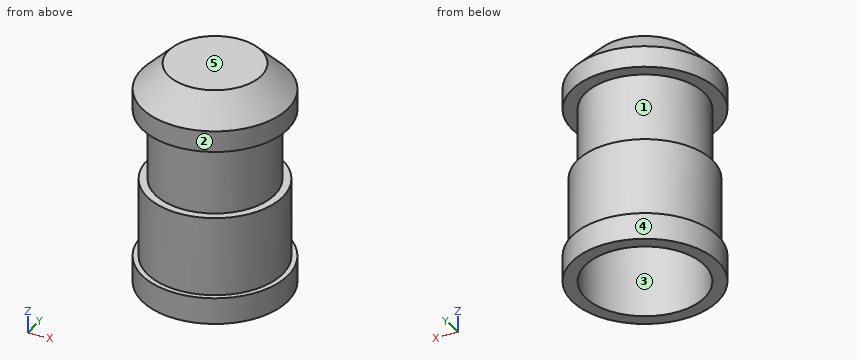
```python
from build123d import *

# Parameters (mm, degrees)
F0_R          = 2.55
F0_R_2        = 2.25
F1_DEPTH      = 4
F2_START      = -3
F0_R_3        = 2.75
F2_DEPTH      = 1
F3_DEPTH      = 4.5
F3_DEPTH_BACK = 1
F4_START      = 2.7
F4_DEPTH      = 1.8
F5_SIZE       = 1


with BuildPart() as f1:
    # F0 (on Top) → F1 (new body)
    with BuildSketch(Plane.XY):
        Circle(F0_R)
        Circle(F0_R_2, mode=Mode.SUBTRACT)
    extrude(amount=-F1_DEPTH)

    # F0 (on Top) → F2 (join)
    with BuildSketch(Plane.XY.offset(F2_START)):
        Circle(F0_R_3)
        Circle(F0_R, mode=Mode.SUBTRACT)
    extrude(amount=-F2_DEPTH)

    # F0 (on Top) → F3 (join, two sides)
    with BuildSketch(Plane.XY) as f3_sk:
        Circle(F0_R_2)
    extrude(amount=F3_DEPTH)
    extrude(f3_sk.sketch, amount=-F3_DEPTH_BACK)

    # F0 (on Top) → F4 (join)
    with BuildSketch(Plane.XY.offset(F4_START)):
        Circle(F0_R_3)
        Circle(F0_R, mode=Mode.SUBTRACT)
        Circle(F0_R)
        Circle(F0_R_2, mode=Mode.SUBTRACT)
    extrude(amount=F4_DEPTH)

    # F5
    f5_edges = [f1.edges().sort_by_distance(p)[0] for p in [
        (-2.75, 0, 4.5),
    ]]
    chamfer(f5_edges, length=F5_SIZE)


solid = f1.part
```
Work out the finished part from the listing and answer in its coordinate system (mm). Face numbers are marked on the shaded views. A direction names the side the tool comes from. Give positions to 0.01 mm unless a question says otherwise; leave off trailing zeros. Write each loop counter-clockwise with the first axis right and the second up, starting at its lowest first coordinate (ties: lowest second). Pieces come first, ordered by that corner, then holes. Notation, with made-up numbers: (-37.75, -40) -> (-28.75, -40) arc R7 ccw to (-28.75, -30) -> close; hole circle Ø7 at (66, -22). An arc over 180 degrees is marked (long way). Write item = value, one per line.
Q1. Section A-A on y = 0 is taken. Determine the outline of the cut face in (x, z), and give its area (4 significant figures).
Computed values:
outline = (-2.75, -4) -> (-2.25, -4) -> (-2.25, -1) -> (2.25, -1) -> (2.25, -4) -> (2.75, -4) -> (2.75, -3) -> (2.55, -3) -> (2.55, 0) -> (2.25, 0) -> (2.25, 2.7) -> (2.75, 2.7) -> (2.75, 3.5) -> (1.75, 4.5) -> (-1.75, 4.5) -> (-2.75, 3.5) -> (-2.75, 2.7) -> (-2.25, 2.7) -> (-2.25, 0) -> (-2.55, 0) -> (-2.55, -3) -> (-2.75, -3) -> close
area = 28.35 mm^2
Q2. A tool of negligible diameter and unlimited length cuts with its end or side. For the marked faces 1 and 2, from which of +Z, -Z, +X, -X, +Y, -Y can it reach the whole face along a straight path? Write none if from no direction.
Computed values:
face_1 = none
face_2 = +Z, -Z
Q3. Section D-D on z = -2 is taken. Determine the outline of the cut face in (x, y), and give its area (3 significant figures).
Computed values:
outline = circle Ø5.1 at (0, 0); hole circle Ø4.5 at (0, 0)
area = 4.52 mm^2
Q4. Section C-C on z = 2.25 is taken. Determine the outline of the cut face in (x, y).
Computed values:
outline = circle Ø4.5 at (0, 0)
Q5. For a pull along Y with two mould halves and no side action, classify the marked faces 3, 4 and 5 as pulls with the +Y half, pulls with the -Y half, needs draft (parallel to the pull), parting line crosses it, or undercut.
Computed values:
face_3 = undercut
face_4 = parting line crosses it
face_5 = needs draft
Q6. Flat-ended cylindrical pins translate along their axes: pin 1 Ø1.3 at (x, y) = (0.5, 0.5) entering from -Z; pin 2 Ø1 at (x, z) = (-2, 3.5) entering from -Y. Find the tip coordinate at first contact, or state that the pin passes through.
Computed values:
pin_1 = -1
pin_2 = -2.3
Q7. Consider line 1 along X through (y, z) = (-0.5, -1.5); line 2 along Y through (x, z) = (0.05, 0.25); line 3 along Z through (x, y) = (2.3, -0.8). Determine where each line is inside the solid, lowest interval first.
Computed values:
line_1 = -2.5 to -2.19, 2.19 to 2.5
line_2 = -2.25 to 2.25
line_3 = -4 to 0, 2.7 to 3.81
